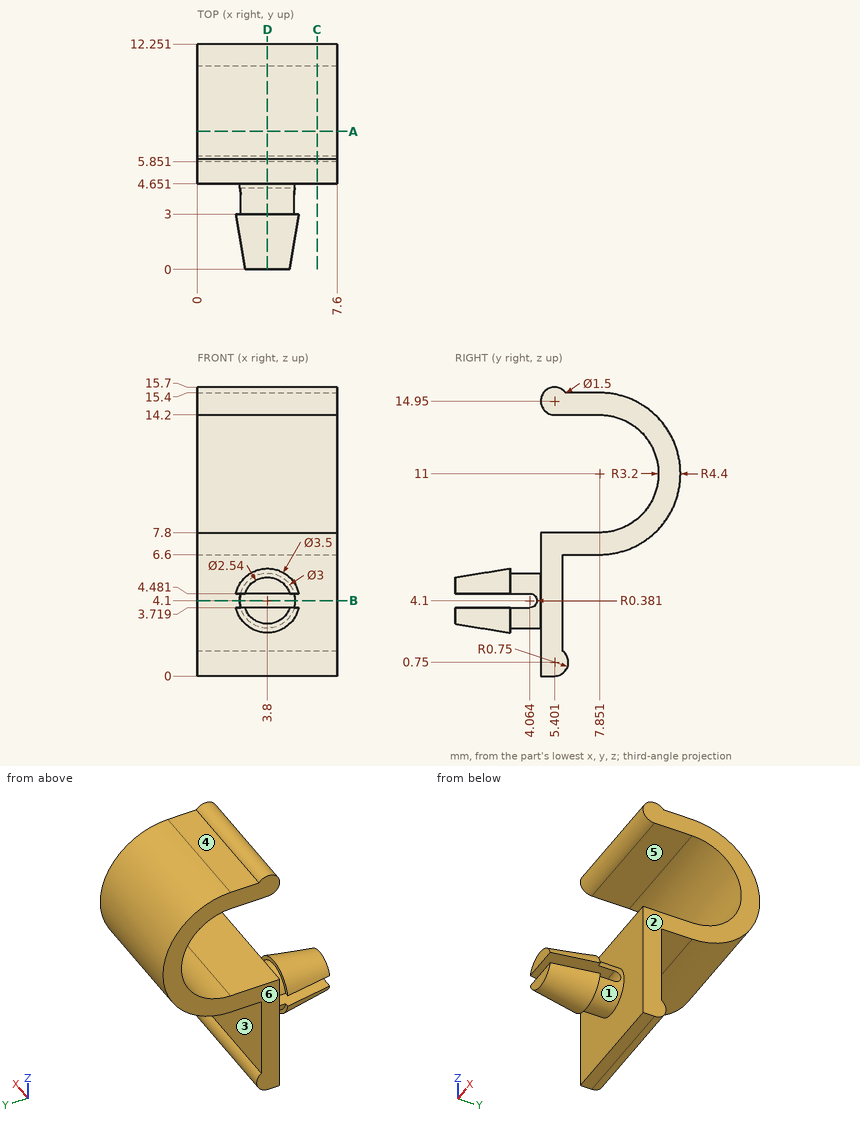
Job drawing, mm, ordinate dimensions from the low corner. One solid piece. A direction names the side the tool comes from. Give positions to 0.01 mm unless a question says otherwise; leave off trailing zeros. Order: outer loops, then holes, each group sorted by start corner. A loop starts at its lowest first (then second) coordinate and runs counter-clockwise, first axis right, second up. Notation, with made-up numbers: (1.5, -19.75) - (49.5, -19.75) arc R22 cw to (49.5, 16.25) - close; hole circle Ø6 at (-16, 36). An arc over 180 degrees is marked (long way). Return JSON: item names as keys, results as strings.
1) Cut at A-A, the plane y = 7.5. Give the cut face in (x, z), plus the area to 3 significant figures.
Geometry says:
{"outline": "(0, 6.6) - (7.6, 6.6) - (7.6, 7.8) - (0, 7.8) - close; (0, 14.2) - (7.6, 14.2) - (7.6, 15.4) - (0, 15.4) - close", "area": "18.2 mm²"}
2) Cut at B-B, the plane z = 4.1. Give the cut face in (x, y) (3 decimals).
Geometry says:
{"outline": "(0, 4.651) - (2.3, 4.651) - (2.3, 4.445) - (5.3, 4.445) - (5.3, 4.651) - (7.6, 4.651) - (7.6, 5.851) - (0, 5.851) - close"}
3) Pull direction Y, two halves, no side cores. Call the marked faces 1, 2 and 3: pulls with the +Y half, pulls with the -Y half, needs draft (parallel to the pull), parting line crosses it, or undercut.
Geometry says:
{"face 1": "undercut", "face 2": "needs draft", "face 3": "pulls with the +Y half"}
4) 3-axis set-ups, long thin cutter, end or side, ignore diameter. For the marked faces 4, 5 and 6: which of +Z, -Z, +X, -X, +Y, -Y reach the whole face in a straight line?
Geometry says:
{"face 4": "+Z, +X, -X, +Y", "face 5": "+X, -X, -Y", "face 6": "+Z, -Z, -X, +Y, -Y"}
5) Flat gauge pins, fed straight in: P1, Ø1.5, axis at x = 4, z = 3, coming from the +Y side; P2, Ø1, axis at x = 4.5, y = 6.5, coming from the -Z side; P3, Ø4, axis at x = 4.5, y = 1, coming from the -Z side; P4, Ø2, axis at y = 9.5, z = 6, coming from the -X side. Where does each tip first touch, or does it go through?
Geometry says:
{"P1": "y = 5.85", "P2": "z = 0.3", "P3": "z = 2.37", "P4": "x = 0"}
6) Probe line 1 (Y direction, x = 5.5, z = 5); line 2 (Z direction, x = 5.25, y = 2.25); line 3 (Z direction, x = 3.25, y = 5.5). List the from-to ranges inside material, lowest first. Write a range as from..to.
Geometry says:
{"line 1": "4.65..5.85", "line 2": "3.36..3.72, 4.48..4.84", "line 3": "0.01..7.8, 14.2..15.69"}
7) Cut at D-D, the plane x = 3.8. Give the cut face in (y, z).
Geometry says:
{"outline": "(0, 2.83) - (3, 2.35) - (3, 2.6) - (4.65, 2.6) - (4.65, 0) - (5.4, 0) arc R0.75 ccw to (5.85, 1.35) - (5.85, 6.6) - (7.85, 6.6) arc R4.4 ccw to (7.85, 15.4) - (6, 15.4) arc R0.75 ccw (long way) to (5.4, 14.2) - (7.85, 14.2) arc R3.2 cw to (7.85, 7.8) - (4.65, 7.8) - (4.65, 5.6) - (3, 5.6) - (3, 5.85) - (0, 5.37) - (0, 4.48) - (4.06, 4.48) arc R0.38 cw to (4.06, 3.72) - (0, 3.72) - close"}
8) Cut at C-C, the plane x = 6.5. Give the cut face in (y, z), plus the area to 3 significant figures.
Geometry says:
{"outline": "(4.65, 0) - (5.4, 0) arc R0.75 ccw to (5.85, 1.35) - (5.85, 6.6) - (7.85, 6.6) arc R4.4 ccw to (7.85, 15.4) - (6, 15.4) arc R0.75 ccw (long way) to (5.4, 14.2) - (7.85, 14.2) arc R3.2 cw to (7.85, 7.8) - (4.65, 7.8) - close", "area": "30.3 mm²"}
